Autodesk Inventor part; units mm, degrees
ref_plane "YZ Plane" through (0, 0, 0) normal (1, 0, 0) x (0, 1, 0)
ref_plane "XZ Plane" through (0, 0, 0) normal (0, 1, 0) x (-1, 0, 0)
ref_plane "XY Plane" through (0, 0, 0) normal (0, 0, 1) x (1, 0, 0)
ref_plane "Work Plane1" through (0, 0, 0) normal (0, 0, 1) x (1, 0, 0)
sketch "Sketch1" plane through (0, 0, 0) normal (0, 0, 1) x (1, 0, 0)
  arc A0 (-15, -23) -> (-13.6245, -24.9) centre (-13, -23) ccw
  line L0 (-13.6245, -24.9) -> (13.6245, -24.9)
  arc A1 (13.6245, -24.9) -> (15, -23) centre (13, -23) ccw
  line L1 (15, -23) -> (15, 23)
  arc A2 (15, 23) -> (13.6245, 24.9) centre (13, 23) ccw
  line L2 (13.6245, 24.9) -> (-13.6245, 24.9)
  arc A3 (-13.6245, 24.9) -> (-15, 23) centre (-13, 23) ccw
  line L3 (-15, 23) -> (-15, -23)
  circle A4 centre (10.5, 13.5) radius 1.4 construction
  circle A5 centre (16.5, 16.5) radius 2.45
  line L4 (-36.2338, -4.8358) -> (15.643, 21.1026)
  line L5 (15.643, 21.1026) -> (19.6679, 13.0528)
  line L6 (19.6679, 13.0528) -> (-32.2089, -12.8856)
  line L7 (-34.8922, -11.9912) -> (-37.1282, -7.519)
  line L8 (-38.0227, -5.7302) -> (19.6679, 13.0528) construction
  line L9 (15.643, 21.1026) -> (-33.9978, -13.78) construction
  line L10 (16.5, 16.5) -> (10.5, 13.5)
  line L11 (16.5, 16.5) -> (19.9213, 18.2106) construction
  line L12 (17.8416, 13.8167) -> (21.2629, 15.5274)
  line L13 (18.5797, 20.8939) -> (15.1584, 19.1833)
  arc A6 (15.1584, 19.1833) -> (17.8416, 13.8167) centre (16.5, 16.5) ccw
  arc A7 (21.2629, 15.5274) -> (18.5797, 20.8939) centre (19.9213, 18.2106) ccw
  arc A8 (-34.8922, -11.9912) -> (-32.2089, -12.8856) centre (-33.1033, -11.0967) ccw
  arc A9 (-36.2338, -4.8358) -> (-37.1282, -7.519) centre (-35.3394, -6.6246) ccw
  circle A10 centre (10.5, 13.5) radius 1.5
  arc A11 (13.5, 9.9688) -> (-21.4758, -7.519) centre (10.6575, -28.0659) ccw
  arc A12 (9.4751, 18.0187) -> (-25.5007, 0.5308) centre (10.6575, -28.0659) ccw
  circle A13 centre (0, -18.9) radius 1.4
  point P0 (0, 0)
  point P1 (-9.1774, 3.6613)
  point P2 (18.2106, 17.3553)
  point P3 (16.3138, 19.761)
  point P4 (18.9971, 14.3944)
  dimension "d0" = 60
  dimension "d1" = 9
  dimension "d2" = 4.5
  dimension "d3" = 8
  dimension "d4" = 6
  dimension "d5" = 2
  dimension "d8" = 3
  dimension "d9" = 14
  dimension "d10" = 14
extrude "Extrusion1" add sketch "Sketch1" along normal blind 3 contours A11 L6 A8 L7 A9 L4 L3 | L3 L4 L1 A6 L6 A11 | L4 A12 L3 | L3 A12 L4 | L1 A6 L12 L5 L6 | L4 L5 L13 A6 L1
fillet "Fillet1" radius 5 4 edges at (-25.5007, 0.5308, 1.5) (-21.4758, -7.519, 1.5) (9.4751, 18.0187, 1.5) (13.5, 9.9688, 1.5)
sketch "Sketch2" plane through (0, 0, 0) normal (0, 0, -1) x (-1, 0, 0)
  circle A0 centre (-10.5, 13.5) radius 1.1933
  circle A1 centre (-10.5, 13.5) radius 1.5
  circle A2 centre (-10.5, 13.5) radius 3
  point P0 (0, 0)
  dimension "d12" = 6
extrude "Extrusion2" add sketch "Sketch2" along normal blind 0.5 contours A2
properties part number "20_Cube_4_insert_xy_levelarm"
CAD build for the part. Positions are in the model's coordinates, mm. A direction names the side the tool comes from. Coordinates: 2 decimals unless noted, no trailing zeros. Loops run counter-clockwise (first coordinate to the right, second up) from the corner with the lowest first, then second, coordinate; pieces in that order, holes last. Notation, with made-up numbers: (34, -15.75) -> (85, -15.75) arc R31 ccw to (85, 23.25) -> close; hole circle Ø3 at (-3.5, 54.5). An arc over 180 degrees is marked (long way). One line per item, written item: value.
1. Which spindle directions (+Z, -Z, +X, -X, +Y, -Y) get a long thin tool onto all of the face, cutting with end or side? Do faces 1 (the face through (15.744, 19.476, 1.479)), 2 (the face through (-33.715, -13.001, 1.479)), 3 (the face through (12.9, 15.3, -0.2)). Say none if no direction does.
Answers:
face 1: +Z, -Z, +X
face 2: +Z, -Z, -Y
face 3: -Z
2. Slice it at C-C on x = -12.5. Write the cut outline in (y, z).
Answers:
outline: (2.24, 0) -> (11.8, 0) -> (11.8, 3) -> (2.24, 3) -> close
3. Slice it at A-A on z = 1.9. Write the cut outline in (x, y), and give its area (3 significant figures).
Answers:
outline: (-37.13, -7.52) -> (-34.89, -11.99) arc R2 ccw to (-32.21, -12.89) -> (-22.67, -8.12) arc R5 ccw to (-20.78, -6.47) arc R38.14 cw to (12.25, 10.04) arc R5 ccw to (14.69, 10.57) -> (19.67, 13.05) -> (19, 14.39) -> (17.84, 13.82) arc R3 cw to (15.16, 19.18) -> (16.31, 19.76) -> (15.64, 21.1) -> (10.44, 18.5) arc R5 cw to (8.45, 17.98) arc R46.1 ccw to (-24.85, 1.33) arc R5 cw to (-26.47, 0.05) -> (-36.23, -4.84) arc R2 ccw to start; hole circle Ø3 at (10.5, 13.5)
area: 481 mm^2
4. Flat gauge pins, fed straight in: P1, Ø5, axis at x = -26.5, y = -0.5, coming from the -Z side; P2, Ø1, axis at x = -29, z = 0.5, coming from the +Y side; P3, Ø1, axis at x = -10.5, z = 1, coming from the -Y side; P4, Ø4, axis at x = 10.5, y = 13.5, coming from the +Z side. Where does each tip first touch, or does it go through?
Answers:
P1: stops at z = 0
P2: stops at y = -0.97
P3: stops at y = 3.33
P4: stops at z = 3
5. Pull direction Y, two halves, no side cores. Call faces 4 (the face through (9, 12, -0.5)), 5 (the face through (13.847, 15.1, 1.479)), 6 (the face through (-6.641, 5.927, 1.479)): pulls with the +Y half, pulls with the -Y half, needs draft (parallel to the pull), parting line crosses it, or undercut.
Answers:
face 4: needs draft
face 5: undercut
face 6: pulls with the -Y half
6. Slice it at B-B on x = -18.5. Write the cut outline in (y, z), and give its area (3 significant figures).
Answers:
outline: (-3.48, 0) -> (7.64, 0) -> (7.64, 3) -> (-3.48, 3) -> close
area: 33.4 mm^2
7. Drill centre lines: line 1 (X direction, y = 14, z = 2.85); line 2 (Z direction, x = -2.5, y = 16); line 3 (Y direction, x = 10.5, z = 0.25). Where is each one in solid material? Low to high. Write a range as [from, to].
Answers:
line 1: x = [-8.2, 9.09], [11.91, 14.84], [18.21, 19.19]
line 2: z = [0, 3]
line 3: y = [10.07, 12], [15, 18.53]
